Build history of the part. All positions in model axes, mm. Face numbers are marked on the shaded views. Round coordinates to 2 decimals unless told otherwise and drop trailing zeros. Loops run counter-clockwise (first coordinate to the right, second up) from the corner with the lowest first, then second, coordinate; pieces in that order, holes last. Notation, with made-up numbers: (-7, 40) -> (-3, 40) arc R16 cw to (-3, 57) -> close; hole circle Ø9 at (8, 64.25). An arc over 180 degrees is marked (long way). Put each result on its own line as item: value. Start each with the question number.
Item 1: Cut at B-B, the plane z = -5.25. List the corners of the cut face in (x, y), plus the area to 3 significant figures.
Item 2: Pull direction X, two halves, no side cores. Call the marked faces 1 and 2: +X half, -X half, draft (parallel to the pull), parting line (faces both ways), or undercut.
Item 3: Flat gauge pins, fed straight in: pin 1 Ø1 at (y, z) = (1.5, 4.5) entering from -X; pin 2 Ø1.5 at (x, y) = (0.5, -2) entering from +Z; pin 3 Ø2 at (x, z) = (-2.5, 7.5) entering from +Y. Where does each tip first touch, or does it go through?
Item 4: Drill centre lines: probe 1 along Y at (x, z) = (0, 3.5); probe 2 along Y at (x, z) = (0.75, 2.75); probe 3 along Z at (x, y) = (-2.5, -3). Where is each one in solid material? Low to high. Write a range as [from, to].
Item 5: Cut at A-A, the plane x = 0. List the corners of the cut face in (y, z).
Item 6: Cut at C-C, the plane y = 3. List the corners of the cut face in (x, z).
```python
from build123d import *

# Parameters (mm, degrees)
ESQUISSE1_R                  = 4
ESQUISSE1_R_2                = 1.25
BOSS_EXTRU_1_DEPTH           = 13
CHANFREIN1_SIZE              = 0.3
ENL_V_MAT_EXTRU_1_DEPTH      = 15.177446879
ENL_V_MAT_EXTRU_1_DEPTH_BACK = 15.177446879
ESQUISSE2_R                  = 3


with BuildPart() as part:
    # Esquisse1 → Boss.-Extru.1 (new, symmetric)
    with BuildSketch(Plane.XY):
        with Locations(Location((0, 0, 0), (0, 0, 180))):
            Circle(ESQUISSE1_R)
        with Locations(Location((0, 0, 0), (0, 0, 180))):
            Circle(ESQUISSE1_R_2, mode=Mode.SUBTRACT)
    extrude(amount=BOSS_EXTRU_1_DEPTH, both=True)

    # Chanfrein1
    chanfrein1_edges = [part.edges().sort_by_distance(p)[0] for p in [
        (4, 0, -13),
        (4, 0, 13),
    ]]
    chamfer(chanfrein1_edges, length=CHANFREIN1_SIZE)

    # Esquisse2 → Enlèv. mat.-Extru.1 (cut, two sides: drawn at the far end of the back side and taken through both)
    with BuildSketch(Plane(origin=(0, 0, 0), x_dir=(1, 0, 0), z_dir=(0, 1, 0)).offset(-ENL_V_MAT_EXTRU_1_DEPTH_BACK)):
        with Locations((0, 13.5)):
            Circle(ESQUISSE2_R)
        with Locations((0, -13.5)):
            Circle(ESQUISSE2_R)
    extrude(amount=ENL_V_MAT_EXTRU_1_DEPTH + ENL_V_MAT_EXTRU_1_DEPTH_BACK, mode=Mode.SUBTRACT)


solid = part.part
```
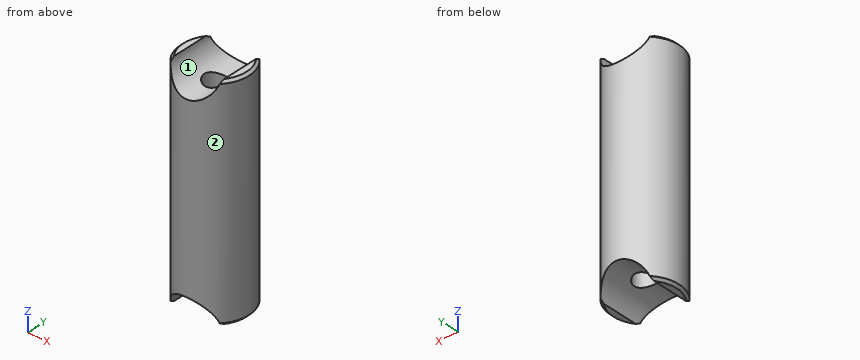
Reply:
1. outline: circle Ø8 at (0, 0); hole circle Ø2.5 at (0, 0)
1. area: 45.4 mm^2
2. face 1: undercut
2. face 2: parting line
3. pin 1: stops at x = -3.87
3. pin 2: stops at z = 10.77
3. pin 3: stops at y = 3.71
4. probe 1: y = [-4, -1.25], [1.25, 4]
4. probe 2: y = [-3.93, -1], [1, 3.93]
4. probe 3: z = [-11.84, 11.84]
5. outline: (-4, -10.5) -> (-1.25, -10.5) -> (-1.25, 10.5) -> (-4, 10.5) -> close; (1.25, -10.5) -> (4, -10.5) -> (4, 10.5) -> (1.25, 10.5) -> close
6. outline: (-2.65, -12.09) arc R3 cw to (2.65, -12.09) -> (2.65, 12.09) arc R3 cw to (-2.65, 12.09) -> close
